from build123d import *

# Parameters (mm, degrees)
F1_DEPTH = 5
F2_R     = 1


with BuildPart() as f1:
    # F0 (on Top) → F1 (new body)
    with BuildSketch(Plane.XY):
        with BuildLine():
            ThreePointArc((-11.324876, -22.119801), (-10.3773, -21.625245), (-9.483998, -22.212185))
            ThreePointArc((-9.483998, -22.212185), (-0.753771, -22.639988), (-5, -15))
            Line((-5, -15), (-6.256602, -15))
            ThreePointArc((-6.256602, -15), (-6.737226, -14.637841), (-6.521601, -14.076001))
            Line((-6.521601, -14.076001), (-2.350005, -11.468753))
            ThreePointArc((-2.350005, -11.468753), (-0.626788, -9.652604), (0, -7.228762))
            Line((0, -7.228762), (0, 0))
            Line((0, 0), (-30, 0))
            Line((-30, 0), (-30, -7.228762))
            ThreePointArc((-30, -7.228762), (-29.373212, -9.652604), (-27.649995, -11.468753))
            Line((-27.649995, -11.468753), (-23.478399, -14.076001))
            ThreePointArc((-23.478399, -14.076001), (-23.262774, -14.637841), (-23.743398, -15))
            Line((-23.743398, -15), (-25, -15))
            ThreePointArc((-25, -15), (-29.246229, -22.639988), (-20.516002, -22.212185))
            ThreePointArc((-20.516002, -22.212185), (-19.6227, -21.625245), (-18.675124, -22.119801))
            Line((-18.675124, -22.119801), (-16.695997, -25.286405))
            ThreePointArc((-16.695997, -25.286405), (-15, -26.226408), (-13.304003, -25.286405))
            Line((-13.304003, -25.286405), (-11.324876, -22.119801))
        make_face()
    extrude(amount=F1_DEPTH)

    # F2
    f2_edges = [f1.edges().sort_by_distance(p)[0] for p in [
        (-29.246229, -22.639988, 5),
    ]]
    fillet(f2_edges, radius=F2_R)


solid = f1.part
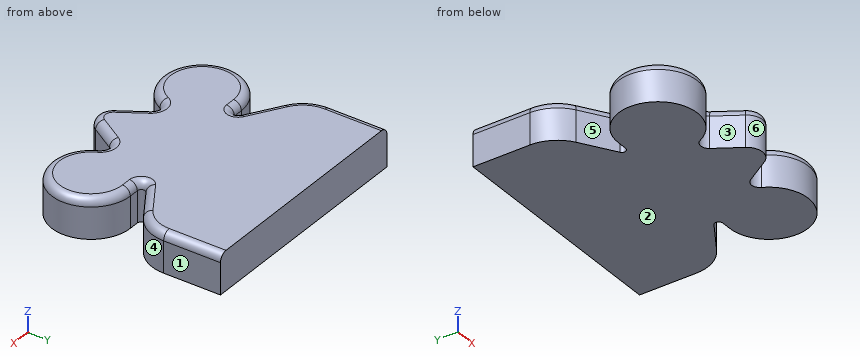
Geometry check sheet. Reference: the model listing, model coordinates, mm. Face numbers are marked on the shaded views. A direction names the side the tool comes from. Give positions to 0.01 mm unless a question says otherwise; leave off trailing zeros. Order: outer loops, then holes, each group sorted by start corner. A loop starts at its lowest first (then second) coordinate and runs counter-clockwise, first axis right, second up.
1) Tool access check on the marked faces 4, 5 and 6. Record the directions out of +Z, -Z, +X, -X, +Y, -Y that give a thin tool (end or side, any length) a straight path to the whole face; none if there is none.
Results are:
face 4: +Z, -Z, +X
face 5: +Z, -Z, -X
face 6: +Z, -Z, -Y
2) Cross-section at B-B (y = -23.5). Give the number of separate pieces and of enclosed holes in the cut face, then the cut area to 3 significant figures.
Results are:
separate pieces: 3
enclosed holes: 0
area: 97.8 mm2
3) Gauge pin test, flat ends, axial feed: pin 1 (2 mm diameter, centred on x = -21.5, z = 4, fed in from -Y); pin 2 (1.5 mm diameter, centred on y = -13, z = 3.5, fed in from +X); pin 3 (3 mm diameter, centred on y = -17, z = 1, fed in from -X). Record the tip position at first contact, or that the pin passes through.
Results are:
pin 1: stops at y = -24.33
pin 2: stops at x = -3.6
pin 3: stops at x = -29.77
4) Draft check along X on the marked faces 1, 2 and 3. Enter one of: released by +X, released by -X, zero draft, split by the parting line, or undercut.
Results are:
face 1: released by +X
face 2: zero draft
face 3: undercut
5) Cross-section at A-A (z = 2.3). Record the boundary of the cut face in (x, y).
Results are:
outline: (-30, -7.23) arc R5 ccw to (-27.65, -11.47) - (-23.48, -14.08) arc R0.5 cw to (-23.74, -15) - (-25, -15) arc R5 ccw (long way) to (-20.52, -22.21) arc R1.06 cw to (-18.68, -22.12) - (-16.7, -25.29) arc R2 ccw to (-13.3, -25.29) - (-11.32, -22.12) arc R1.06 cw to (-9.48, -22.21) arc R5 ccw (long way) to (-5, -15) - (-6.26, -15) arc R0.5 cw to (-6.52, -14.08) - (-2.35, -11.47) arc R5 ccw to (0, -7.23) - (0, 0) - (-30, 0) - close
6) Material ranges on probe 1 along X at (y, z) = (-21.75, 2.55); probe 2 along X at (y, z) = (-22, 0.3); probe 3 along Y at (x, z) = (-19.5, 2.85), recorded low to high.
Results are:
probe 1: x = -29.68 to -20.07, -19.07 to -10.93, -9.93 to -0.32
probe 2: x = -29.58 to -20.38, -18.76 to -11.24, -9.62 to -0.42
probe 3: y = -21.63 to 0
